Check sheet for the modelled part. Datum: model origin and axes. Units: mm. A direction names the side the tool comes from. Coordinates: 2 decimals unless noted, no trailing zeros. Loops run counter-clockwise (first coordinate to the right, second up) from the corner with the lowest first, then second, coordinate; pieces in that order, holes last. Notation, with made-up numbers: M 33.5,-36 L 39.5,-36 A28 cw 39.5,-6 Z; hole C -3,80.5 d1. An arc over 180 degrees is marked long. Return JSON: item names as keys, results as strings.
from build123d import *

# Parameters (mm, degrees)
F0_R      = 20
F1_DEPTH  = 50
F2_DEPTH  = 2.5
F4_W      = 40
F4_H      = 50
F5_DEPTH  = 25
F6_W      = 8
F6_H      = 28.5657137142
F7_DEPTH  = 2.5
F8_DEPTH  = 50
F3_R      = 17.5
F9_DEPTH  = 50
F11_DEPTH = 25
F12_R     = 1


with BuildPart() as f1:
    # F0 (on Top) → F1 (new body)
    with BuildSketch(Plane.XY):
        Circle(F0_R)
    extrude(amount=F1_DEPTH)

    # F2 (add): a face of the model
    f2_faces = [f1.faces().sort_by_distance(p)[0] for p in [
        (0, 0, 0),
    ]]
    extrude(f2_faces, amount=F2_DEPTH)

    # F4 (on Front) → F5 (cut, symmetric)
    with BuildSketch(Plane.XZ):
        with Locations((6, 37.5)):
            Rectangle(F4_W, F4_H)
    extrude(amount=F5_DEPTH, both=True, mode=Mode.SUBTRACT)

    # F6 (on Top) → F7 (join)
    with BuildSketch(Plane.XY):
        with Locations((-18, 0)):
            Rectangle(F6_W, F6_H)
    extrude(amount=-F7_DEPTH)

    # F6 (on Top) → F8 (join)
    with BuildSketch(Plane.XY):
        with Locations((-18, 0)):
            Rectangle(F6_W, F6_H)
    extrude(amount=F8_DEPTH)

    # F3 (on Top) → F9 (cut)
    with BuildSketch(Plane.XY):
        Circle(F3_R)
    extrude(amount=F9_DEPTH, mode=Mode.SUBTRACT)

    # F10 (on Right) → F11 (cut)
    with BuildSketch(Plane.YZ):
        with BuildLine():
            Line((8.25, 17.3), (8.25, 50.5))
            Line((8.25, 50.5), (-8.25, 50.5))
            Line((-8.25, 50.5), (-8.25, 17.3))
            ThreePointArc((-8.25, 17.3), (-7.8964466094, 17.1535533906), (-7.75, 16.8))
            ThreePointArc((-7.75, 16.8), (-7.8964466094, 16.4464466094), (-8.25, 16.3))
            Line((-8.25, 16.3), (-8.25, 5.5))
            Line((-8.25, 5.5), (8.25, 5.5))
            Line((8.25, 5.5), (8.25, 16.3))
            ThreePointArc((8.25, 16.3), (7.75, 16.8), (8.25, 17.3))
        make_face()
    extrude(amount=-F11_DEPTH, mode=Mode.SUBTRACT)

    # F12
    f12_edges = [f1.edges().sort_by_distance(p)[0] for p in [
        (20, 0, -2.5),
        (-18, 14.282857, -2.5),
        (-22, 0, -2.5),
        (-18, -14.282857, -2.5),
        (-14, -14.282857, 5),
        (-14, 14.282857, 5),
        (-22, 14.282857, 23.75),
        (-22, -14.282857, 23.75),
        (-14.759599, -9.402352, 50),
        (-14, -12.391428, 50),
        (-18, -14.282857, 50),
        (-22, -11.266428, 50),
        (-18.716662, -8.25, 50),
        (-14, 12.391428, 50),
        (-14.759599, 9.402352, 50),
        (-18.716662, 8.25, 50),
        (-22, 11.266428, 50),
        (-18, 14.282857, 50),
    ]]
    fillet(f12_edges, radius=F12_R)


solid = f1.part
1) Scan lines: line 1 along Y through (x, z) = (-15.5, 19); line 2 along Z through (x, y) = (-9, 8.5); line 3 along X through (y, z) = (-10.5, 5). Record each from-to range of solid material in increasing order. Write a range as [from, to].
Answers:
{"line 1": "[-14.28, -8.25], [8.25, 14.28]", "line 2": "[-2.5, 0]", "line 3": "[-22, -14], [14, 17.02]"}
2) Go/stop test with flat-tipped pins: pin 1 Ø3.5 at (x, z) = (-17.5, 33.5) entering from +Y; pin 2 Ø7 at (x, z) = (-18.5, 32) entering from -Y; pin 3 Ø7 at (x, y) = (-20, -3) entering from +Z. Record where each tip stops, or that it passes through.
Answers:
{"pin 1": "y = 14.28", "pin 2": "y = -14.28", "pin 3": "z = 5.5"}
3) Draft check along Y on faces 5 (the face through (-18, 11, 50)), 6 (the face through (-18, 14.283, 23)), 7 (the face through (-19, -8.25, 11)), 8 (the face through (-19, 8.25, 33)). Enter one of: +Y half, -Y half, draft (parallel to the pull), parting line (faces both ways), or undercut.
Answers:
{"face 5": "draft", "face 6": "+Y half", "face 7": "undercut", "face 8": "undercut"}
4) Set-up check for faces 1 (the face through (17, -6, 12.5)), 2 (the face through (17.41, 1.78, 6.24)), 3 (the face through (-19, 8.25, 11)), 4 (the face through (-19, -8.25, 33)): record each of +Z, -Z, +X, -X, +Y, -Y from which the full face is reachable in a straight line by a thin tool's end or side.
Answers:
{"face 1": "+Z, +X, +Y, -Y", "face 2": "+Z", "face 3": "-X", "face 4": "+Z, +X, -X"}
5) Section check B-B on x = 0. Record the cut outline in (y, z).
Answers:
{"outline": "M -20,-1.5 A1 ccw -19,-2.5 L 19,-2.5 A1 ccw 20,-1.5 L 20,12.5 L 17.5,12.5 L 17.5,0 L -17.5,0 L -17.5,12.5 L -20,12.5 Z"}
6) Section check A-A on z = 24. Record the cut outline in (x, y), then the cut area to 3 significant figures.
Answers:
{"outline": "M -22,-13.28 A1 ccw -21,-14.28 L -14,-14.28 L -14,-10.5 A17.5 cw -15.43,-8.25 L -22,-8.25 Z; M -22,8.25 L -15.43,8.25 A17.5 cw -14,10.5 L -14,14.28 L -21,14.28 A1 ccw -22,13.28 Z", "area": "92.7 mm²"}
